from build123d import *

# Parameters (mm, degrees)
SKETCH001_R     = 25.8969
PAD001_DEPTH    = 15
SKETCH004_R     = 30.1625
PAD002_DEPTH    = 3
SKETCH002_R     = 15.1
POCKET_DEPTH    = 9
SKETCH003_R     = 13
POCKET001_DEPTH = 15.001


with BuildPart() as part:
    # Sketch001 → Pad001 (new body)
    with BuildSketch(Plane.XY):
        Circle(SKETCH001_R)
    extrude(amount=PAD001_DEPTH)

    # Sketch004 → Pad002 (join)
    with BuildSketch(Plane.XY.offset(15)):
        Circle(SKETCH004_R)
    extrude(amount=-PAD002_DEPTH)

    # Sketch002 → Pocket (cut)
    with BuildSketch(Plane.XY.offset(15)):
        Circle(SKETCH002_R)
    extrude(amount=-POCKET_DEPTH, mode=Mode.SUBTRACT)

    # Sketch003 → Pocket001 (cut, through all)
    with BuildSketch(Plane.XY):
        Circle(SKETCH003_R)
    extrude(amount=POCKET001_DEPTH, mode=Mode.SUBTRACT)


solid = part.part
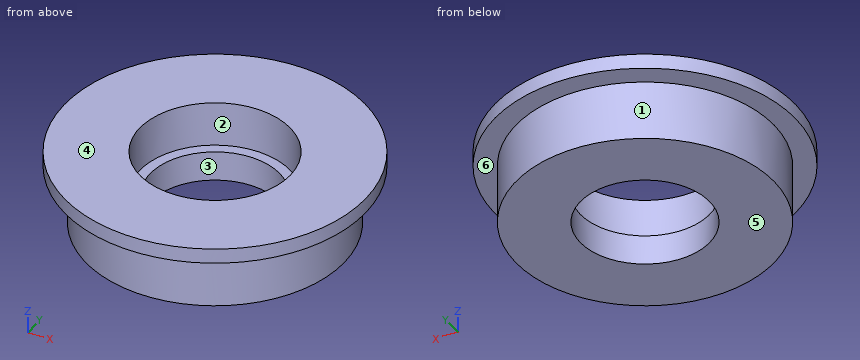
Could you check a few things on this model? Use its own coordinates, in mm. Face numbers are marked on the shaded views. A direction names the side the tool comes from. Coordinates: 2 decimals unless noted, no trailing zeros. Loops run counter-clockwise (first coordinate to the right, second up) from the corner with the lowest first, then second, coordinate; pieces in that order, holes last.
1. We'd pull the mould along Y, two halves only. Please class the marked faces 1, 2, 3 and 4: released by +Y, released by -Y, zero draft, split by the parting line, or undercut.
2. For the marked faces 5 and 6, which set-ups out of +Z, -Z, +X, -X, +Y, -Y let a thin tool reach every point of the face, with its end or its side?
3. For P1, Ø6, axis at x = 13, z = 7.5, coming from the -Y side; P2, Ø1, axis at x = 5, z = 8, coming from the +Y side; P3, Ø6, axis at y = 9.5, z = 2.5, coming from the -X side, each with a flat end and sliding along its axis, tell me the tip position at first contact or that it passes through.
4. Imagine slicing it at A-A (y = 0). Please give me the cut outline in (x, z), and give its area (3 significant figures).
5. Imagine slicing it at C-C (z = 10). Please give me the cut outline in (x, y), and give its area (3 significant figures).
6. Imagine slicing it at D-D (y = -19). Please give me the cut outline in (x, z), and give its area (3 significant figures).
7. I need wall thicknesses on L1, parallel to X at y = 0, z = 3.8; L2, parallel to Z at x = -4.5, y = -14. Which ranges of each line are inside material? Lowest first, please.
Computed values:
1. face 1: split by the parting line
1. face 2: undercut
1. face 3: undercut
1. face 4: zero draft
2. face 5: -Z, +X, -X, +Y, -Y
2. face 6: -Z
3. P1: stops at y = -23.89
3. P2: stops at y = 25.5
3. P3: stops at x = -25.07
4. outline: (-30.16, 12) - (-25.9, 12) - (-25.9, 0) - (-13, 0) - (-13, 6) - (-15.1, 6) - (-15.1, 15) - (-30.16, 15) - close; (13, 0) - (25.9, 0) - (25.9, 12) - (30.16, 12) - (30.16, 15) - (15.1, 15) - (15.1, 6) - (13, 6) - close
4. area: 375 mm2
5. outline: circle Ø51.79 at (0, 0); hole circle Ø30.2 at (0, 0)
5. area: 1,390 mm2
6. outline: (-23.43, 12) - (-17.6, 12) - (-17.6, 0) - (17.6, 0) - (17.6, 12) - (23.43, 12) - (23.43, 15) - (-23.43, 15) - close
6. area: 563 mm2
7. L1: x = -25.9 to -13, 13 to 25.9
7. L2: z = 0 to 6
